For this review, take the finished solid that the model builds, in its own axes (mm). Give positions to 0.01 mm unless a question says otherwise; leave off trailing zeros. Loops run counter-clockwise (first coordinate to the right, second up) from the corner with the lowest first, then second, coordinate; pieces in that order, holes last. Notation, with made-up numbers: (35.5, -36.75) - (67.5, -36.75) arc R31 ccw to (67.5, -5.75) - close; hole circle Ø6 at (-20.5, 83.25). An arc over 180 degrees is marked (long way). Put each result on its own line as item: value.
from build123d import *

# Parameters (mm, degrees)
SKETCH_1_W          = 30
SKETCH_1_H          = 30
SKETCH_1_R          = 14.5
EXTRUDE_1_DEPTH     = 10
FILLET_1_R          = 2
SKETCH_2_R          = 1.5
CUT_EXTRUDE_1_DEPTH = 10


with BuildPart() as part:
    # 草圖1 → 填料-伸長1 (new body)
    with BuildSketch(Plane.XY):
        Rectangle(SKETCH_1_W, SKETCH_1_H)
        Circle(SKETCH_1_R, mode=Mode.SUBTRACT)
    extrude(amount=EXTRUDE_1_DEPTH)

    # 圓角1
    fillet_1_edges = [part.edges().sort_by_distance(p)[0] for p in [
        (-15, 15, 5),
        (15, 15, 5),
        (15, -15, 5),
        (-15, -15, 5),
    ]]
    fillet(fillet_1_edges, radius=FILLET_1_R)

    # 草圖2 → 除料-伸長1 (cut)
    with BuildSketch(Plane.XY.offset(10)):
        with Locations((-12, 12)):
            Circle(SKETCH_2_R)
        with Locations(Location((12, 12, 0), (0, 0, 180))):
            Circle(SKETCH_2_R)
        with Locations((12, -12)):
            Circle(SKETCH_2_R)
        with Locations(Location((-12, -12, 0), (0, 0, 180))):
            Circle(SKETCH_2_R)
    extrude(amount=-CUT_EXTRUDE_1_DEPTH, mode=Mode.SUBTRACT)


solid = part.part
1) Wall thickness on line 1 (X direction, y = 11, z = 8.5); line 2 (Y direction, x = -12, z = 3.25); line 3 (Y direction, x = 0, z = 7): over which ranges is each line inside the solid? List them lowest first.
Geometry check:
line 1: x = -15 to -13.12, -10.88 to -9.45, 9.45 to 10.88, 13.12 to 15
line 2: y = -15 to -13.5, -10.5 to -8.14, 8.14 to 10.5, 13.5 to 15
line 3: y = -15 to -14.5, 14.5 to 15
2) Take a section at C-C on z = 3.5. State the section outline as (x, y) points.
Geometry check:
outline: (-15, -13) arc R2 ccw to (-13, -15) - (13, -15) arc R2 ccw to (15, -13) - (15, 13) arc R2 ccw to (13, 15) - (-13, 15) arc R2 ccw to (-15, 13) - close; hole circle Ø29 at (0, 0); hole circle Ø3 at (-12, -12); hole circle Ø3 at (-12, 12); hole circle Ø3 at (12, -12); hole circle Ø3 at (12, 12)
3) Take a section at D-D on x = 12. State the section outline as (y, z) points, and give its area (3 significant figures).
Geometry check:
outline: (-15, 0) - (-13.5, 0) - (-13.5, 10) - (-15, 10) - close; (-10.5, 0) - (-8.14, 0) - (-8.14, 10) - (-10.5, 10) - close; (8.14, 0) - (10.5, 0) - (10.5, 10) - (8.14, 10) - close; (13.5, 0) - (15, 0) - (15, 10) - (13.5, 10) - close
area: 77.2 mm²
4) Insertion check: pin 1 Ø3.5 at (x, y) = (-12, -12) entering from +Z. The pin has a flat end and moves straight along its axis. Give the tip position at first contact, or say it passes through.
Geometry check:
pin 1: stops at z = 10
5) Take a section at B-B on y = 0. State the section outline as (x, z) points.
Geometry check:
outline: (-15, 0) - (-14.5, 0) - (-14.5, 10) - (-15, 10) - close; (14.5, 0) - (15, 0) - (15, 10) - (14.5, 10) - close
6) Take a section at A-A on x = -10. State the section outline as (y, z) points.
Geometry check:
outline: (-15, 0) - (-10.5, 0) - (-10.5, 10) - (-15, 10) - close; (10.5, 0) - (15, 0) - (15, 10) - (10.5, 10) - close
7) Draft analysis for pull direction Y (two halves, no side actions). For faces 1 (the face through (6.691, -12.864, 4.93)), 2 (the face through (2.2, 14.5, 0)), 3 (the face through (-14.43, 14.4, 5.07)), state which applies: pulls with the +Y half, pulls with the -Y half, needs draft (parallel to the pull), parting line crosses it, or undercut.
Geometry check:
face 1: undercut
face 2: needs draft
face 3: pulls with the +Y half
